```python
from build123d import *

# Parameters (mm, degrees)
CHAMFER1_SIZE = 0.508


with BuildPart() as part:
    # Sketch1 → Revolve1 (revolve)
    with BuildSketch(Plane.XY):
        Polygon((-3.175, 47.0723), (-3.175, 57.15), (0, 57.15), (0, 0), (-3.175, 0), (-3.175, 8.2357), (-2.667, 8.2357), (-2.667, 8.9723), (-3.175, 8.9723), (-3.175, 21.1389), (-2.667, 21.1389), (-2.667, 21.8755), (-3.175, 21.8755), (-3.175, 46.3357), (-2.667, 46.3357), (-2.667, 47.0723), align=None)
    revolve(axis=Axis((0, 0, 0), (0, -1, 0)))

    # Chamfer1
    chamfer1_edges = [part.edges().sort_by_distance(p)[0] for p in [
        (3.175, 0, 0),
        (3.175, 57.15, 0),
    ]]
    chamfer(chamfer1_edges, length=CHAMFER1_SIZE)


solid = part.part
```
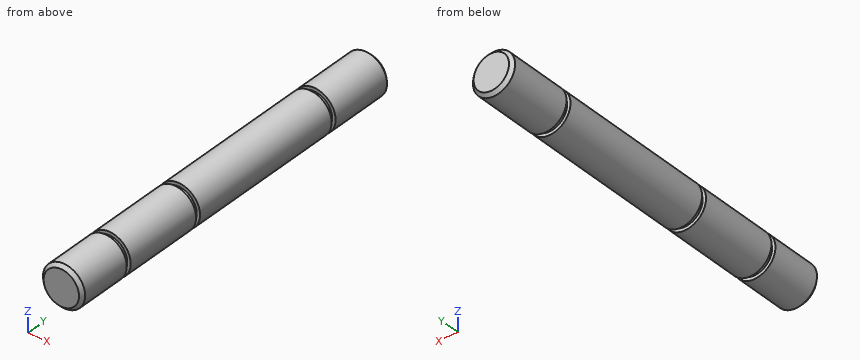
Verification items for the finished model (mm, model axes). Coordinates: 2 decimals unless noted, no trailing zeros. Write each loop counter-clockwise with the first axis right and the second up, starting at its lowest first coordinate (ties: lowest second). Pieces come first, ordered by that corner, then holes. Notation, with made-up numbers: (59.25, 27) - (92.25, 27) arc R13 cw to (92.25, 41) - close; hole circle Ø4 at (74.5, -21.75). An arc over 180 degrees is marked (long way). Write item = value, one per line.
Q1. Cross-section at A-A (y = 22.5). Enter the section's corners in (x, z) (3 decimals), plus the area to 3 significant figures.
Answer:
outline = circle Ø6.35 at (0, 0)
area = 31.7 mm²
Q2. Go/stop test with a flat-tipped pin: pin 1 Ø2 at (x, z) = (2, 1) entering from -Y. Record where the tip stops, or that it passes through.
Answer:
pin_1 = 0
Q3. Material ranges on L1, parallel to Y at x = 2.5, z = 1.25; L2, parallel to Y at x = -2.5, z = -1.5; L3, parallel to Z at x = -0.25, y = 25.5, recorded low to high. Write a range as from..to.
Answer:
L1 = 0.13..8.24, 8.97..21.14, 21.88..46.34, 47.07..57.02
L2 = 0.25..8.24, 8.97..21.14, 21.88..46.34, 47.07..56.9
L3 = -3.17..3.17
